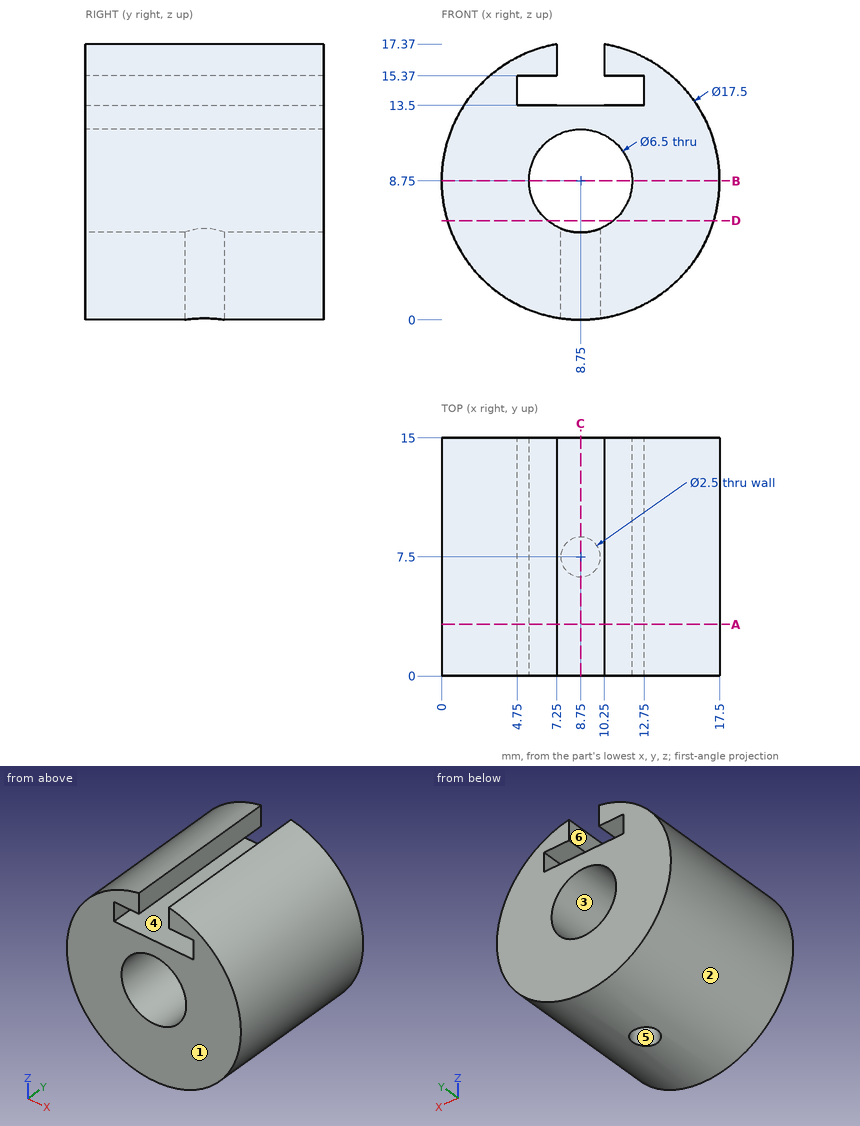
Geometry: see drawing. Coordinates: mm, zero at the bounding-box minimum. A direction names the side the tool comes from. Give positions to 0.01 mm unless a question says otherwise; leave off trailing zeros. Order: outer loops, then holes, each group sorted by start corner. A loop starts at its lowest first (then second) coordinate and runs counter-clockwise, first axis right, second up. Notation, with made-up numbers: (60.25, 13) - (90.25, 13) arc R25 cw to (90.25, 35) - close; hole circle Ø6 at (-24, 69). An arc over 180 degrees is marked (long way). Use a Markdown table: item, result.
(1) Section query C-C (x = 8.75). Output: boundary loops of the cut face in (y, z).
Computed values:
| item | result |
|---|---|
| outline | (0, 0) - (6.25, 0) - (6.25, 5.5) - (0, 5.5) - close; (0, 12) - (15, 12) - (15, 13.5) - (0, 13.5) - close; (8.75, 0) - (15, 0) - (15, 5.5) - (8.75, 5.5) - close |
(2) Section query B-B (z = 8.75). Output: boundary loops of the cut face in (x, y), then the cut area to 3 significant figures.
Computed values:
| item | result |
|---|---|
| outline | (0, 0) - (5.5, 0) - (5.5, 15) - (0, 15) - close; (12, 0) - (17.5, 0) - (17.5, 15) - (12, 15) - close |
| area | 165 mm2 |
(3) Access query for the marked faces 4, 5 and 6. Directions: +Z, -Z, +X, -X, +Y, -Y. A direction counts if a zero-diameter tool reaches every point of the face in a straight line with its end or side. Return the directions, or none.
Computed values:
| item | result |
|---|---|
| face 4 | +Y, -Y |
| face 5 | -Z |
| face 6 | +Z, +Y, -Y |
(4) Section query A-A (y = 3.25). Output: boundary loops of the cut face in (x, z).
Computed values:
| item | result |
|---|---|
| outline | (4.75, 13.5) - (4.75, 15.37) - (7.25, 15.37) - (7.25, 17.37) arc R8.75 ccw (long way) to (10.25, 17.37) - (10.25, 15.37) - (12.75, 15.37) - (12.75, 13.5) - close; hole circle Ø6.5 at (8.75, 8.75) |
(5) Line query: line 1 (Y direction, x = 8.75, z = 2.2); line 2 (Z direction, x = 8.75, y = 10.75); line 3 (Z direction, x = 5.75, y = 1.25) (1 decimal). Output: solid intervals per line, ascending. Write a range as from..to.
Computed values:
| item | result |
|---|---|
| line 1 | y = 0..6.25, 8.75..15 |
| line 2 | z = 0..5.5, 12..13.5 |
| line 3 | z = 0.5..7.5, 10..13.5, 15.4..17 |
(6) Pin query (flat end, axial travel): pin 1 (8 mm diameter, centred on y = 13, z = 4.5, fed in from +X); pin 2 (1 mm diameter, centred on y = 8, z = 17, fed in from +X) (1 decimal); pin 3 (2 mm diameter, centred on x = 12, y = 9, fed in from +Z) (1 decimal). Return the tip coordinate at first contact, or that it passes through.
Computed values:
| item | result |
|---|---|
| pin 1 | stops at x = 17.5 |
| pin 2 | stops at x = 12.8 |
| pin 3 | stops at z = 17.2 |
(7) Draft query along Z for the marked faces 1, 2 and 3. Return one class per face: released by +Z, released by -Z, zero draft, split by the parting line, or undercut.
Computed values:
| item | result |
|---|---|
| face 1 | zero draft |
| face 2 | split by the parting line |
| face 3 | undercut |
(8) Section query D-D (z = 6.25). Output: boundary loops of the cut face in (x, y) (1 decimal).
Computed values:
| item | result |
|---|---|
| outline | (0.4, 0) - (6.7, 0) - (6.7, 15) - (0.4, 15) - close; (10.8, 0) - (17.1, 0) - (17.1, 15) - (10.8, 15) - close |
